Geometry check sheet. Reference: drawing and pictorial views, mm from the part's lowest x, y, z. A direction names the side the tool comes from. Give positions to 0.01 mm unless a question says otherwise; leave off trailing zeros. Order: outer loops, then holes, each group sorted by start corner. A loop starts at its lowest first (then second) coordinate and runs counter-clockwise, first axis right, second up. Notation, with made-up numbers: (29.5, 48) - (40.5, 48) arc R4 cw to (40.5, 54) - close; hole circle Ø3 at (3.25, 60). An arc over 180 degrees is marked (long way). Answer in a Markdown table with one row per item.
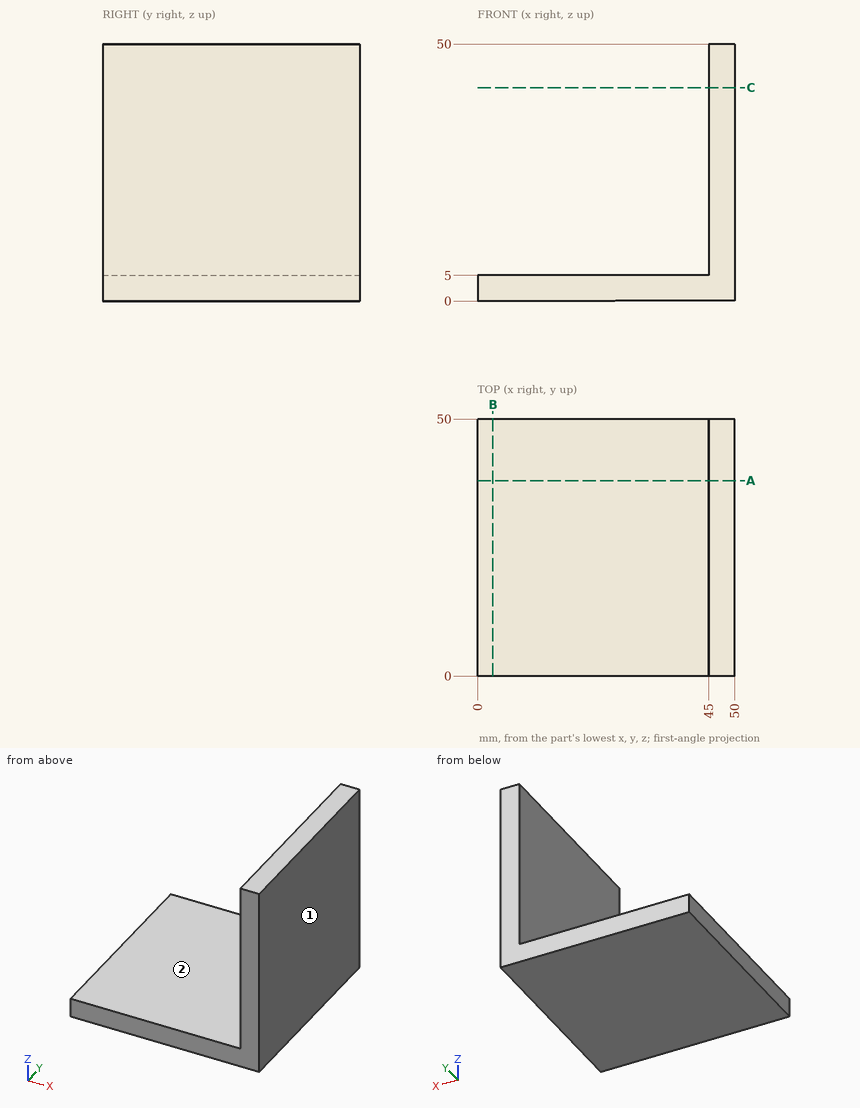
(1) Cross-section at A-A, the plane y = 38. Record the cut outline in (x, z).
Geometry says:
| item | result |
|---|---|
| outline | (0, 0) - (50, 0) - (50, 50) - (45, 50) - (45, 5) - (0, 5) - close |
(2) Gauge pin test, flat end, axial feed: P1, Ø5, axis at y = 23, z = 8, coming from the -X side. Record the tip position at first contact, or that the pin passes through.
Geometry says:
| item | result |
|---|---|
| P1 | x = 45 |
(3) Cross-section at B-B, the plane x = 3. Record the cut outline in (y, z), then the cut area to 3 significant figures.
Geometry says:
| item | result |
|---|---|
| outline | (0, 0) - (50, 0) - (50, 5) - (0, 5) - close |
| area | 250 mm² |
(4) Cross-section at C-C, the plane z = 41.5. Record the cut outline in (x, y), then the cut area to 3 significant figures.
Geometry says:
| item | result |
|---|---|
| outline | (45, 0) - (50, 0) - (50, 50) - (45, 50) - close |
| area | 250 mm² |
(5) Thickness scan on L1, parallel to X at y = 35, z = 44.5; L2, parallel to Z at x = 7.5, y = 37. Record the ranges inside material, lowest first.
Geometry says:
| item | result |
|---|---|
| L1 | 45 to 50 |
| L2 | 0 to 5 |
(6) Access from +Z, -Z, +X, -X, +Y, -Y to the whole of each face (thin tool, end or side, straight path). Record for the marked faces 1 and 2.
Geometry says:
| item | result |
|---|---|
| face 1 | +Z, -Z, +X, +Y, -Y |
| face 2 | +Z, -X, +Y, -Y |
